The model under review builds one solid part; all positions refer to its coordinate system, in mm. Face numbers are marked on the shaded views. Coordinates: 2 decimals unless noted, no trailing zeros. Order: outer loops, then holes, each group sorted by start corner. A loop starts at its lowest first (then second) coordinate and runs counter-clockwise, first axis right, second up. Notation, with made-up numbers: M 25.5,2.5 L 57.5,2.5 A31 cw 57.5,37.5 Z; hole C 15,-15.5 d2. An arc over 180 degrees is marked long. Write each question's results on one line, items separated by ' | '.
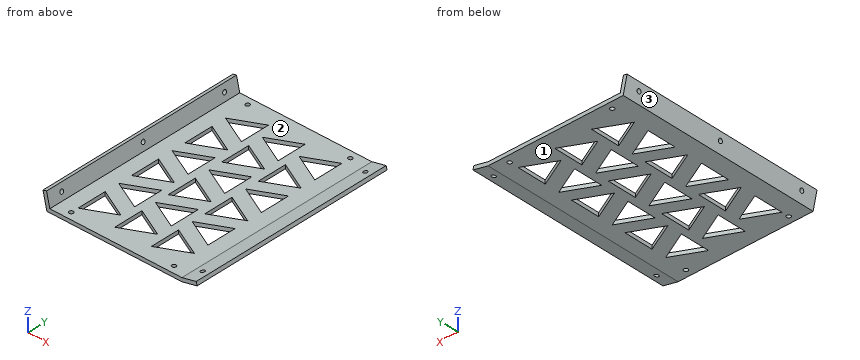
from build123d import *

# Parameters (mm, degrees)
SKETCH1_W              = 114.3
SKETCH1_H              = 177.8
BOSS_EXTRUDE1_DEPTH    = 3.175
BOSS_EXTRUDE2_DEPTH    = 177.8
SKETCH3_R              = 1.778
CUT_EXTRUDE1_DEPTH     = 203.2
CUT_EXTRUDE2_DEPTH     = 3.175
LPATTERN2_COUNT        = 3
LPATTERN2_PITCH        = 50
LPATTERN3_COUNT        = 3
LPATTERN3_PITCH        = 31.75
LPATTERN3_COPY_1_DEPTH = 3.175
LPATTERN3_COPY_2_DEPTH = 3.175
LPATTERN3_COPY_3_DEPTH = 3.175
LPATTERN3_COPY_4_DEPTH = 3.175
SKETCH5_R              = 1.778
CUT_EXTRUDE3_DEPTH     = 3.175
SKETCH6_R              = 1.778
CUT_EXTRUDE4_DEPTH     = 3.175


with BuildPart() as part:
    # Sketch1 → Boss-Extrude1 (new body)
    with BuildSketch(Plane.XY):
        with Locations((-57.15, -88.9)):
            Rectangle(SKETCH1_W, SKETCH1_H)
    extrude(amount=BOSS_EXTRUDE1_DEPTH)

    # Sketch2 → Boss-Extrude2 (add)
    with BuildSketch(Plane.XZ.offset(177.8)):
        Polygon((-114.3, 3.175), (-117.087804878, 15.565243902), (-120.185365854, 14.868292683), (-116.84, 0), (-114.3, 0), align=None)
        Polygon((0, 3.175), (0, 0), (13.087195122, 2.865243902), (12.390243902, 5.962804878), align=None)
    extrude(amount=-BOSS_EXTRUDE2_DEPTH)

    # Sketch3 → Cut-Extrude1 (cut)
    with BuildSketch(Plane(origin=(-108.112433076, 0, -24.325297442), x_dir=(0.219512195, 0, -0.975609756), z_dir=(0.975609756, 0, 0.219512195))):
        with Locations((-34.537804878, -165.1)):
            Circle(SKETCH3_R)
        with Locations((-34.537804878, -88.9)):
            Circle(SKETCH3_R)
        with Locations((-34.537804878, -12.7)):
            Circle(SKETCH3_R)
    extrude(amount=-CUT_EXTRUDE1_DEPTH, mode=Mode.SUBTRACT)

    # Sketch4 → Cut-Extrude2 (cut)
    with BuildSketch(Plane.XY.offset(3.175)):
        Polygon((-101.6, -165.1), (-101.6, -139.7), (-76.2, -152.4), align=None)
        Polygon((-101.6, -127), (-76.2, -139.7), (-76.2, -114.3), align=None)
    cut_extrude2 = extrude(amount=-CUT_EXTRUDE2_DEPTH, mode=Mode.SUBTRACT)

    # LPattern2: Cut-Extrude2 ×3
    with Locations(*[(0, i * LPATTERN2_PITCH, 0) for i in range(1, LPATTERN2_COUNT)]):
        add(cut_extrude2, mode=Mode.SUBTRACT)

    # LPattern3: Cut-Extrude2 ×3
    with Locations(*[(i * LPATTERN3_PITCH, 0, 0) for i in range(1, LPATTERN3_COUNT)]):
        add(cut_extrude2, mode=Mode.SUBTRACT)

    # LPattern3 copy 1 sketch → LPattern3 copy 1 (cut)
    with BuildSketch(Plane(origin=(31.75, 50, 3.175), x_dir=(1, 0, 0), z_dir=(0, 0, 1))):
        Polygon((-101.6, -165.1), (-101.6, -139.7), (-76.2, -152.4), align=None)
        Polygon((-101.6, -127), (-76.2, -139.7), (-76.2, -114.3), align=None)
    extrude(amount=-LPATTERN3_COPY_1_DEPTH, mode=Mode.SUBTRACT)

    # LPattern3 copy 2 sketch → LPattern3 copy 2 (cut)
    with BuildSketch(Plane(origin=(63.5, 50, 3.175), x_dir=(1, 0, 0), z_dir=(0, 0, 1))):
        Polygon((-101.6, -165.1), (-101.6, -139.7), (-76.2, -152.4), align=None)
        Polygon((-101.6, -127), (-76.2, -139.7), (-76.2, -114.3), align=None)
    extrude(amount=-LPATTERN3_COPY_2_DEPTH, mode=Mode.SUBTRACT)

    # LPattern3 copy 3 sketch → LPattern3 copy 3 (cut)
    with BuildSketch(Plane(origin=(31.75, 100, 3.175), x_dir=(1, 0, 0), z_dir=(0, 0, 1))):
        Polygon((-101.6, -165.1), (-101.6, -139.7), (-76.2, -152.4), align=None)
        Polygon((-101.6, -127), (-76.2, -139.7), (-76.2, -114.3), align=None)
    extrude(amount=-LPATTERN3_COPY_3_DEPTH, mode=Mode.SUBTRACT)

    # LPattern3 copy 4 sketch → LPattern3 copy 4 (cut)
    with BuildSketch(Plane(origin=(63.5, 100, 3.175), x_dir=(1, 0, 0), z_dir=(0, 0, 1))):
        Polygon((-101.6, -165.1), (-101.6, -139.7), (-76.2, -152.4), align=None)
        Polygon((-101.6, -127), (-76.2, -139.7), (-76.2, -114.3), align=None)
    extrude(amount=-LPATTERN3_COPY_4_DEPTH, mode=Mode.SUBTRACT)

    # Sketch5 → Cut-Extrude3 (cut)
    with BuildSketch(Plane.XY.offset(3.175)):
        with Locations((-101.6, -171.45)):
            Circle(SKETCH5_R)
        with Locations((-12.7, -171.45)):
            Circle(SKETCH5_R)
        with Locations((-12.7, -6.35)):
            Circle(SKETCH5_R)
        with Locations((-101.6, -6.35)):
            Circle(SKETCH5_R)
    extrude(amount=-CUT_EXTRUDE3_DEPTH, mode=Mode.SUBTRACT)

    # Sketch6 → Cut-Extrude4 (cut)
    with BuildSketch(Plane(origin=(-0.679952409, 0, 3.022010708), x_dir=(0.975609756, 0, 0.219512195), z_dir=(-0.219512195, 0, 0.975609756))):
        with Locations((7.04695122, -165.1)):
            Circle(SKETCH6_R)
        with Locations((7.04695122, -12.7)):
            Circle(SKETCH6_R)
    extrude(amount=-CUT_EXTRUDE4_DEPTH, mode=Mode.SUBTRACT)


solid = part.part
1) The part is to be moulded in two halves that separate along X. For the marked faces 1, 2 and 3, say which applies: pulls with the +X half, pulls with the -X half, needs draft (parallel to the pull), parting line crosses it, or undercut.
Solutions:
face 1: needs draft | face 2: undercut | face 3: pulls with the -X half
2) Take a section at C-C on y = -72. State the section outline as (x, z) points (3 decimals), plus the area to 3 significant figures.
Solutions:
outline: M -120.185,14.868 L -116.84,0 L -91.6,0 L -91.6,3.175 L -114.3,3.175 L -117.088,15.565 Z; M -76.2,0 L -59.85,0 L -59.85,3.175 L -76.2,3.175 Z; M -44.45,0 L -28.1,0 L -28.1,3.175 L -44.45,3.175 Z; M -12.7,0 L 0,0 L 13.087,2.865 L 12.39,5.963 L 0,3.175 L -12.7,3.175 Z | area: 306 mm2
3) Take a section at B-B on y = -156.5. State the section outline as (x, z) points (3 decimals).
Solutions:
outline: M -120.185,14.868 L -116.84,0 L -101.6,0 L -101.6,3.175 L -114.3,3.175 L -117.088,15.565 Z; M -84.4,0 L -69.85,0 L -69.85,3.175 L -84.4,3.175 Z; M -52.65,0 L -38.1,0 L -38.1,3.175 L -52.65,3.175 Z; M -20.9,0 L 0,0 L 13.087,2.865 L 12.39,5.963 L 0,3.175 L -20.9,3.175 Z
4) For pin 1 (3 mm diameter, centred on y = -23.5, z = 6, fed in from -X); pin 2 (3 mm diameter, centred on x = -101.6, y = -6.35, fed in from +Z); pin 3 (1.6 mm diameter, centred on y = -23.5, z = 1, fed in from -X) (3 decimals); pin 4 (2.5 mm diameter, centred on y = -50.5, z = 2.5, fed in from +X), all flat-tipped, find the tip position at first contact; note any pin that passes through.
Solutions:
pin 1: x = -118.53 | pin 2: through | pin 3: x = -117.245 | pin 4: x = 13.09
5) Take a section at A-A on x = -25.5. State the section outline as (y, z) points (3 decimals), plus the area to 3 significant figures.
Solutions:
outline: M -177.8,0 L -158.8,0 L -158.8,3.175 L -177.8,3.175 Z; M -146,0 L -133.3,0 L -133.3,3.175 L -146,3.175 Z; M -120.7,0 L -108.8,0 L -108.8,3.175 L -120.7,3.175 Z; M -96,0 L -83.3,0 L -83.3,3.175 L -96,3.175 Z; M -70.7,0 L -58.8,0 L -58.8,3.175 L -70.7,3.175 Z; M -46,0 L -33.3,0 L -33.3,3.175 L -46,3.175 Z; M -20.7,0 L 0,0 L 0,3.175 L -20.7,3.175 Z | area: 323 mm2
6) To check wall thickness, follow line 1 along Z through (x, y) = (-11, -151.5) (3 decimals); line 2 along Y through (x, z) = (-12, 2.25); line 3 along Z through (x, y) = (7, -142). State the ranges of each line that lie inside material, in increasing order.
Solutions:
line 1: 0 to 3.175 | line 2: -177.8 to -173.08, -169.82 to -7.98, -4.72 to 0 | line 3: 1.53 to 4.75
